```python
from build123d import *

# Parameters (mm, degrees)
F0_W     = 33.3
F0_H     = 12.7
F1_DEPTH = 52
F3_DEPTH = 12.7
F4_R     = 4
F5_DEPTH = 46.001
F6_R     = 3.571875
F7_DEPTH = 25
F8_R     = 3.571875
F9_DEPTH = 25
F10_R    = 10


with BuildPart() as f1:
    # F0 (on Top) → F1 (new body)
    with BuildSketch(Plane.XY):
        with Locations((16.65, -6.35)):
            Rectangle(F0_W, F0_H)
        Polygon((46, 0), (33.3, 0), (33.3, -12.7), (33.3, -46), (46, -46), align=None)
    extrude(amount=F1_DEPTH)

    # F2 (on face) → F3 (join)
    with BuildSketch(Plane.XY.offset(52)):
        Polygon((46, -46), (46, 0), (0, 0), (0, -12.7), (8.125442, -20.825442), (25.174558, -37.874558), (33.3, -46), align=None)
        with BuildLine():
            Line((25.174558, -37.874558), (8.125442, -20.825442))
            ThreePointArc((8.125442, -20.825442), (10.344245, -35.655755), (25.174558, -37.874558))
        make_face()
    extrude(amount=-F3_DEPTH)

    # F4 (on face) → F5 (cut, through all)
    with BuildSketch(Plane.YZ.offset(46)):
        with Locations((-32, 25)):
            Circle(F4_R)
    extrude(amount=-F5_DEPTH, mode=Mode.SUBTRACT)

    # F6 (on face) → F7 (cut)
    with BuildSketch(Plane(origin=(0, 0, 0), x_dir=(-1, 0, 0), z_dir=(0, 1, 0))):
        with Locations((-13, 25.4)):
            Circle(F6_R)
    extrude(amount=-F7_DEPTH, mode=Mode.SUBTRACT)

    # F8 (on face) → F9 (cut)
    with BuildSketch(Plane.XY.offset(52)):
        with Locations((20.119892, -25.880108)):
            Circle(F8_R)
    extrude(amount=-F9_DEPTH, mode=Mode.SUBTRACT)

    # F10
    f10_edges = [f1.edges().sort_by_distance(p)[0] for p in [
        (39.65, -46, 0),
        (0, -6.35, 0),
    ]]
    fillet(f10_edges, radius=F10_R)


solid = f1.part
```
Design review of the part built by this model. Coordinates are the model's own, in mm. A direction names the side the tool comes from. Coordinates: 2 decimals unless noted, no trailing zeros. Write each loop counter-clockwise with the first axis right and the second up, starting at its lowest first coordinate (ties: lowest second). Pieces come first, ordered by that corner, then holes.
1) Insertion check: pin 1 (4 mm diameter, centred on x = 26, z = 17, fed in from -Y); pin 2 (13 mm diameter, centred on y = -32, z = 25, fed in from -X). Each pin has a flat end and moves straight along its axis. Give the tip position at first contact, or say it passes through.
2) Add section C-C (z = 22.5). Write out the cut boundary in (x, y), plus the area to 3 significant figures.
3) Add section D-D (y = -17). Write out the cut boundary in (x, z), plus the area to 3 significant figures.
4) To check wall thickness, follow L1, parallel to X at y = -30.5, z = 9; L2, parallel to Y at x = 3, z = 19.5; L3, parallel to Z at x = 13, y = -6. State the ranges of each line that lie inside material, in increasing order.
5) Add section B-B (y = -23). Write out the cut boundary in (x, z), plus the area to 3 significant figures.
6) Add section A-A (x = 13). Write out the cut boundary in (y, z).
7) Mouldability with a two-part tool opening along X and no side actions: class faces 1 (the cylindrical face through (19.65, -22.34, 45.74)), 2 (the cylindrical face through (2.85, -6.26, 3.01)), 3 (the cylindrical face through (10.19, -35.5, 45.74)), 4 (the flat face through (28, -18, 52)) as +X half, -X half, draft (parallel to the pull), parting line (faces both ways), or undercut.
8) Machinability: for faces 5 (the flat face through (40, -46, 31)), 6 (the flat face through (20, -22, 39.3)), 7 (the flat face through (23, 0, 26)), 8 (the flat face through (29.2, -41.9, 45.7)), 9 (the flat face through (4, -16.7, 45.7)), which of the approach directions +Z, -Z, +X, -X, +Y, -Y give a long, thin tool a straight path to every point of the face, cutting with its end or side? Answer none if there is none.
Check result:
1. pin 1: stops at y = -12.7
1. pin 2: stops at x = 33.3
2. outline: (0, -12.7) - (10.91, -12.7) - (10.91, 0) - (0, 0) - close; (15.09, -12.7) - (33.3, -12.7) - (33.3, -28.88) - (46, -28.88) - (46, 0) - (15.09, 0) - close; (33.3, -46) - (46, -46) - (46, -35.12) - (33.3, -35.12) - close
2. area: 875 mm2
3. outline: (4.3, 39.3) - (33.3, 39.3) - (33.3, 0) - (46, 0) - (46, 52) - (4.3, 52) - close
3. area: 1,030 mm2
4. L1: x = 33.3 to 46
4. L2: y = -12.7 to 0
4. L3: z = 0 to 21.83, 28.97 to 52
5. outline: (7.22, 39.3) - (18.01, 39.3) - (18.01, 52) - (7.22, 52) - close; (22.23, 39.3) - (33.3, 39.3) - (33.3, 0) - (46, 0) - (46, 52) - (22.23, 52) - close
5. area: 938 mm2
6. outline: (-37.68, 39.3) - (-12.7, 39.3) - (-12.7, 28.97) - (0, 28.97) - (0, 52) - (-37.68, 52) - close; (-12.7, 0) - (0, 0) - (0, 21.83) - (-12.7, 21.83) - close
7. face 1: undercut
7. face 2: -X half
7. face 3: undercut
7. face 4: draft
8. face 5: +Z, -Z, +X, -X, -Y
8. face 6: -Z, -X, -Y
8. face 7: +Z, -Z, +X, -X, +Y
8. face 8: +Z, -Z, -Y
8. face 9: +Z, -Z, -X
